from build123d import *

# Parameters (mm, degrees)
F1_DEPTH     = 25.4
F2_T         = -2.54
F4_D         = 22.86
F6_D         = 22.86
F9_T1_DEPTH  = 63.2859311747
F9_T3_DEPTH  = 63.2859311747
F9_T5_DEPTH  = 63.2859311747
F9_T7_DEPTH  = 63.2859311747
F9_T9_DEPTH  = 63.2859311747
F9_T11_DEPTH = 63.2859311747
F9_T13_DEPTH = 63.2859311747


# Not quite as in the source:
# - a fillet or chamfer that OpenCascade refuses, or shapes differently, is made with other operations: its cross-section is extruded or revolved along the edge and cut away or added
# - the program builds the solid bodies; features that only make, move or delete a surface that nothing else refers to are left out


with BuildPart() as f1:
    # F0 (on Top) → F1 (new body)
    with BuildSketch(Plane.XY):
        Polygon((27.2259101757, 34.1301219533), (-9.7089265027, 42.5658566882), (-39.3327434985, 18.9486331517), (-39.3382023982, -18.9372976297), (-9.721192539, -42.5630570455), (27.2160735783, -34.1379663779), (43.6590811844, -0.0062907401), align=None)
    extrude(amount=F1_DEPTH)

    # F2
    f2_openings = [f1.faces().sort_by_distance(p)[0] for p in [
        (0, 0, 25.4),
    ]]
    offset(amount=F2_T, openings=f2_openings)

    # F4 (through all)
    with Locations(Plane.XY.offset(2.54)):
        with Locations((-12.0702767901, -5.8105965731)):
            Hole(F4_D / 2)

    # F6 (through all)
    with Locations(Plane.XY.offset(2.54)):
        with Locations((7.7538759853, 10.4717538884)):
            Hole(F6_D / 2)

    # F9: fillet of radius 5.08 on 7 edges, made by hand

    # F9_s2 → F9_t1 (cut)
    with BuildSketch(Plane(origin=(30.848595501, -7.0456672344, 0), x_dir=(0, 0, 1), z_dir=(-0.9748958395, 0.2226614068, 0))):
        with BuildLine():
            ThreePointArc((25.4, 34.2554733567), (23.9121024484, 37.8475758051), (20.32, 39.3354733567))
            Line((20.32, 39.3354733567), (25.4, 39.3354733567))
            Line((25.4, 39.3354733567), (25.4, 34.2554733567))
        make_face()
    extrude(amount=F9_T1_DEPTH, mode=Mode.SUBTRACT)

    # F9_s4 → F9_t3 (cut)
    with BuildSketch(Plane(origin=(24.7423091554, 19.7255014847, 0), x_dir=(0, 0, 1), z_dir=(-0.7819213116, -0.623377143, 0))):
        with BuildLine():
            ThreePointArc((25.4, 34.2554733567), (23.9121024484, 37.8475758051), (20.32, 39.3354733567))
            Line((20.32, 39.3354733567), (25.4, 39.3354733567))
            Line((25.4, 39.3354733567), (25.4, 34.2554733567))
        make_face()
    extrude(amount=F9_T3_DEPTH, mode=Mode.SUBTRACT)

    # F9_s6 → F9_t5 (cut)
    with BuildSketch(Plane(origin=(0.0045593646, 31.6429652589, 0), x_dir=(0, 0, 1), z_dir=(-0.0001440878, -0.9999999896, 0))):
        with BuildLine():
            ThreePointArc((25.4, 34.2554733567), (23.9121024484, 37.8475758051), (20.32, 39.3354733567))
            Line((20.32, 39.3354733567), (25.4, 39.3354733567))
            Line((25.4, 39.3354733567), (25.4, 34.2554733567))
        make_face()
    extrude(amount=F9_T5_DEPTH, mode=Mode.SUBTRACT)

    # F9_s8 → F9_t7 (cut)
    with BuildSketch(Plane(origin=(-24.7366237207, 19.7326307943, 0), x_dir=(0, 0, 1), z_dir=(0.7817416371, -0.6236024477, 0))):
        with BuildLine():
            ThreePointArc((25.4, 34.2554733567), (23.9121024484, 37.8475758051), (20.32, 39.3354733567))
            Line((20.32, 39.3354733567), (25.4, 39.3354733567))
            Line((25.4, 39.3354733567), (25.4, 34.2554733567))
        make_face()
    extrude(amount=F9_T7_DEPTH, mode=Mode.SUBTRACT)

    # F9_s10 → F9_t9 (cut)
    with BuildSketch(Plane(origin=(-30.8506246092, -7.0367771307, 0), x_dir=(0, 0, 1), z_dir=(0.9749599646, 0.2223804564, 0))):
        with BuildLine():
            ThreePointArc((20.32, 39.3354733567), (23.9121024484, 37.8475758051), (25.4, 34.2554733567))
            Line((25.4, 34.2554733567), (25.4, 39.3354733567))
            Line((25.4, 39.3354733567), (20.32, 39.3354733567))
        make_face()
    extrude(amount=F9_T9_DEPTH, mode=Mode.SUBTRACT)

    # F9_s12 → F9_t11 (cut)
    with BuildSketch(Plane(origin=(-13.7334759289, -28.5073483522, 0), x_dir=(0, 0, 1), z_dir=(0.4340135532, 0.9009063412, 0))):
        with BuildLine():
            ThreePointArc((20.32, 39.3354733567), (23.9121024484, 37.8475758051), (25.4, 34.2554733567))
            Line((25.4, 34.2554733567), (25.4, 39.3354733567))
            Line((25.4, 39.3354733567), (20.32, 39.3354733567))
        make_face()
    extrude(amount=F9_T11_DEPTH, mode=Mode.SUBTRACT)

    # F9_s14 → F9_t13 (cut)
    with BuildSketch(Plane(origin=(13.7252602377, -28.5113048206, 0), x_dir=(0, 0, 1), z_dir=(-0.433753916, 0.9010313759, 0))):
        with BuildLine():
            ThreePointArc((20.32, 39.3354733567), (23.9121024484, 37.8475758051), (25.4, 34.2554733567))
            Line((25.4, 34.2554733567), (25.4, 39.3354733567))
            Line((25.4, 39.3354733567), (20.32, 39.3354733567))
        make_face()
    extrude(amount=F9_T13_DEPTH, mode=Mode.SUBTRACT)


solid = f1.part
The model under review builds one solid part; all positions refer to its coordinate system, in mm. A direction names the side the tool comes from. Round coordinates to 2 decimals unless told otherwise and drop trailing zeros. Write each loop counter-clockwise with the first axis right and the second up, starting at its lowest first coordinate (ties: lowest second). Pieces come first, ordered by that corner, then holes. Notation, with made-up numbers: (44.25, -14) - (48.25, -14) arc R11 ccw to (48.25, 7) - close; hole circle Ø9 at (21.5, 74). An arc over 180 degrees is marked (long way). One line per item, written item: value. Start each with the question number.
1. The part is to be moulded in two halves that separate along Y. For faces 1 (the face through (8.49, -38.41, 10.02)), 2 (the face through (35.56, 16.82, 10.02)), 3 (the face through (33.26, 15.74, 13.47)), say which applies: released by +Y, released by -Y, zero draft, split by the parting line, or undercut.
2. Consider section B-B on y = 2. State how many separate pieces and enclosed holes the cut face has, and give its area (3 significant figures).
3. Consider section A-A on z = 19. Write out the cut boundary in (x, y).
4. Clearance check with flat-ended pins moving along their axes: P1, Ø1, axis at y = 27, z = 14, coming from the +X side; P2, Ø1, axis at y = 30, z = 19, coming from the -X side; P3, Ø1, axis at x = -29.5, z = 10.5, coming from the +Y side; P4, Ø13.5, axis at x = -12.07, y = -5.81, coming from the +Z side. State where each tip first meets the part, or that it passes through.
5. Machinability: for faces 4 (the face through (9.02, 38.29, 10.02)), 5 (the face through (-22.74, 28.93, 13.47)), which of the approach directions +Z, -Z, +X, -X, +Y, -Y give a long, thin tool a straight path to every point of the face, cutting with its end or side? Answer none if there is none.
6. To check wall thickness, follow L1, parallel to Z at x = -32, y = 21; L2, parallel to X at y = 31, z = 20.25; L3, parallel to Y at x = 40, z = 17.25. State the ranges of each line that lie inside material, in increasing order. Write a range as from..to.
Checks:
1. face 1: released by -Y
1. face 2: released by +Y
1. face 3: undercut
2. separate pieces: 3
2. enclosed holes: 0
2. area: 239 mm^2
3. outline: (-39.34, -18.94) - (-9.72, -42.56) - (27.22, -34.14) - (43.66, -0.01) - (27.23, 34.13) - (-9.71, 42.57) - (-39.33, 18.95) - close; hole (-36.8, -17.71) - (-9.09, -39.81) - (25.46, -31.93) - (40.84, -0.01) - (25.47, 31.93) - (-9.08, 39.82) - (-36.79, 17.73) - close
4. P1: stops at x = 30.9
4. P2: stops at x = -26.1
4. P3: stops at y = 27.19
4. P4: passes through
5. face 4: +Z, -Z, +X, +Y
5. face 5: +Z
6. L1: z = 0..2.54
6. L2: x = -24.22..-20.14, 25.91..28.73
6. L3: y = -7.6..-1.75, 1.74..7.59
